Here's how the part is built. I have some questions about the finished solid (model axes, mm). Coordinates: 2 decimals unless noted, no trailing zeros. Write each loop counter-clockwise with the first axis right and the second up, starting at its lowest first coordinate (ties: lowest second). Pieces come first, ordered by that corner, then holes.
```python
from build123d import *

# Parameters (mm, degrees)
SKETCH_1_R      = 2
SKETCH_1_R_2    = 13.25
SKETCH_1_R_3    = 2.5
EXTRUDE_1_DEPTH = 4
FILLET_1_R      = 5
CHAMFER_1_SIZE  = 0.5


with BuildPart() as part:
    # 草图1 → 凸台-拉伸1 (new body)
    with BuildSketch(Plane.XY):
        with BuildLine():
            Line((-27, 0), (-27, 70))
            Line((-27, 70), (-11.999997176, 70))
            Line((-11.999997176, 70), (22.879375353, 14.336463423))
            ThreePointArc((22.879375353, 14.336463423), (7.458447073, -25.949403987), (-27, 0))
        make_face()
        with Locations((-22, 60)):
            Circle(SKETCH_1_R, mode=Mode.SUBTRACT)
        with Locations((-22, 50)):
            Circle(SKETCH_1_R, mode=Mode.SUBTRACT)
        with Locations((-22, 30)):
            Circle(SKETCH_1_R, mode=Mode.SUBTRACT)
        with Locations((-22, 40)):
            Circle(SKETCH_1_R, mode=Mode.SUBTRACT)
        with Locations((-12, 50)):
            Circle(SKETCH_1_R, mode=Mode.SUBTRACT)
        Circle(SKETCH_1_R_2, mode=Mode.SUBTRACT)
        with Locations((-12, 40)):
            Circle(SKETCH_1_R, mode=Mode.SUBTRACT)
        with Locations((-19, 14)):
            Circle(SKETCH_1_R_3, mode=Mode.SUBTRACT)
    extrude(amount=EXTRUDE_1_DEPTH)

    # 圆角1
    fillet_1_edges = [part.edges().sort_by_distance(p)[0] for p in [
        (-11.999997176, 70, 2),
    ]]
    fillet(fillet_1_edges, radius=FILLET_1_R)

    # 倒角1
    chamfer_1_edges = [part.edges().sort_by_distance(p)[0] for p in [
        (-27, 70, 2),
    ]]
    chamfer(chamfer_1_edges, length=CHAMFER_1_SIZE)


solid = part.part
```
1) Imagine slicing it at D-D on y = -4.5. Please give me the cut outline in (x, z).
Values follow:
outline: (-26.62, 0) - (-12.46, 0) - (-12.46, 4) - (-26.62, 4) - close; (12.46, 0) - (26.62, 0) - (26.62, 4) - (12.46, 4) - close
2) Will these pins go through, and if not, where does the flat tip stop? pin 1 (2.5 mm diameter, centred on x = -12, y = 40, fed in from +Z); pin 2 (1.5 mm diameter, centred on y = 43, z = 3, fed in from +X); pin 3 (6.5 mm diameter, centred on x = -12, y = 50, fed in from -Z); pin 4 (2 mm diameter, centred on x = 13.5, z = 2, fed in from -Y).
Values follow:
pin 1: passes through
pin 2: stops at x = 5.39
pin 3: stops at z = 0
pin 4: stops at y = -23.93
3) Imagine slicing it at B-B on y = 50. Please give me the cut outline in (x, z), then the cut area to 3 significant figures.
Values follow:
outline: (-27, 0) - (-24, 0) - (-24, 4) - (-27, 4) - close; (-20, 0) - (-14, 0) - (-14, 4) - (-20, 4) - close; (-10, 0) - (0.53, 0) - (0.53, 4) - (-10, 4) - close
area: 78.1 mm2
4) Imagine slicing it at A-A on z = 2.55. Count the separate pieces of the cut face and the enclosed holes in it, then the cut area to 3 significant figures.
Values follow:
separate pieces: 1
enclosed holes: 8
area: 3,060 mm2
5) We'd pull the mould along Y, two halves only. Please class faces 1 (the face through (8.128, -25.747, 1.972)), 2 (the face through (7.123, 11.172, 1.972)), 3 (the face through (-21, 70, 2)): pulls with the +Y half, pulls with the -Y half, needs draft (parallel to the pull), parting line crosses it, or undercut.
Values follow:
face 1: parting line crosses it
face 2: undercut
face 3: pulls with the +Y half
6) Imagine slicing it at C-C on x = -18.5. Please give me the cut outline in (y, z), then the cut area to 3 significant figures.
Values follow:
outline: (-19.67, 0) - (11.55, 0) - (11.55, 4) - (-19.67, 4) - close; (16.45, 0) - (70, 0) - (70, 4) - (16.45, 4) - close
area: 339 mm2
7) I need wall thicknesses on probe 1 along Y at (x, z) = (-22, 1.1); probe 2 along X at (y, z) = (13.5, 1.7); probe 3 along X at (y, z) = (-5, 0.65). Which ranges of each line are inside material? Lowest first, please.
Values follow:
probe 1: y = -15.65 to 28, 32 to 38, 42 to 48, 52 to 58, 62 to 70
probe 2: x = -27 to -21.45, -16.55 to 23.38
probe 3: x = -26.53 to -12.27, 12.27 to 26.53
